from build123d import *

# Parameters (mm, degrees)
F0_W     = 650
F0_H     = 20
F1_DEPTH = 20
F3_D     = 9
F4_W     = 365
F4_H     = 20
F4_R     = 4.5
F5_DEPTH = 25


with BuildPart() as f1:
    # F0 (on Top) → F1 (new body)
    with BuildSketch(Plane.XY):
        with Locations((-0.1587718725, -31.5417255368)):
            Rectangle(F0_W, F0_H)
    extrude(amount=F1_DEPTH)

    # F3 (through all)
    with Locations(Plane.XY.offset(20)):
        with Locations((-245.1587718725, -31.5417255368), (-151.8187718725, -31.5417255368), (-46.8287718725, -31.5417255368), (46.5112281275, -31.5417255368)):
            Hole(F3_D / 2)

    # F4 (on face) → F5 (cut)
    with BuildSketch(Plane.XY.offset(20)):
        with Locations((142.3412281275, -31.5417255368)):
            Rectangle(F4_W, F4_H)
        with Locations((46.5112281275, -31.5417255368)):
            Circle(F4_R, mode=Mode.SUBTRACT)
    extrude(amount=-F5_DEPTH, mode=Mode.SUBTRACT)


solid = f1.part
Build history of the part. All positions in model axes, mm. Give positions to 0.01 mm unless a question says otherwise; leave off trailing zeros. Loops run counter-clockwise (first coordinate to the right, second up) from the corner with the lowest first, then second, coordinate; pieces in that order, holes last. Notation, with made-up numbers: (75.25, 27.5) - (89.25, 27.5) arc R29 cw to (89.25, 58.5) - close; hole circle Ø9 at (27.5, 33). An arc over 180 degrees is marked (long way). Write item = value, one per line. Start each with the question number.
1) Pull direction Y, two halves, no side cores. Call faces 1 (the cylindrical face through (-240.663, -31.344, 9.86)), 2 (the flat face through (-185, -31, 0)), 3 (the cylindrical face through (-148.5, -28.5, 9.9)), 4 (the flat face through (-185, -41.542, 10)): +Y half, -Y half, draft (parallel to the pull), parting line (faces both ways), or undercut.
2) Probe probe 1 along X at (y, z) = (-32, 1.25); probe 2 along X at (y, z) = (-31.25, 10.5). List the from-to ranges inside material, lowest first. Write a range as from..to.
3) Band-saw the part on A-A on z = 16. Give the cut face in (x, y).
Final values:
q1.face_1 = undercut
q1.face_2 = draft
q1.face_3 = undercut
q1.face_4 = -Y half
q2.probe_1 = -325.16..-249.64, -240.68..-156.3, -147.34..-51.31, -42.35..-40.16
q2.probe_2 = -325.16..-249.65, -240.67..-156.31, -147.33..-51.32, -42.34..-40.16
q3.outline = (-325.16, -41.54) - (-40.16, -41.54) - (-40.16, -21.54) - (-325.16, -21.54) - close; hole circle Ø9 at (-245.16, -31.54); hole circle Ø9 at (-151.82, -31.54); hole circle Ø9 at (-46.83, -31.54)
